The listing builds one solid part. Answer for the finished solid, in the listing's coordinates (mm). Face numbers are marked on the shaded views. A direction names the side the tool comes from. Coordinates: 2 decimals unless noted, no trailing zeros. Write each loop counter-clockwise with the first axis right and the second up, starting at its lowest first coordinate (ties: lowest second). Pieces come first, ordered by that corner, then holes.
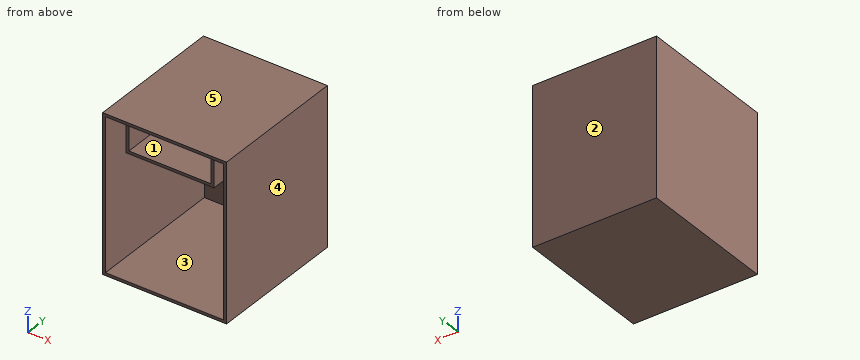
from build123d import *

# Parameters (mm, degrees)
F0_W     = 831.85
F0_H     = 1054.1
F0_W_2   = 793.75
F0_H_2   = 1016
F1_DEPTH = 914.4
F2_W     = 831.85
F2_H     = 1054.1
F3_DEPTH = 19.05
F6_DEPTH = 406.4


with BuildPart() as f1:
    # F0 (on Front) → F1 (new body)
    with BuildSketch(Plane.XZ):
        with Locations((396.875, 508)):
            Rectangle(F0_W, F0_H)
        with Locations((396.875, 508)):
            Rectangle(F0_W_2, F0_H_2, mode=Mode.SUBTRACT)
    extrude(amount=-F1_DEPTH)

    # F2 (on face) → F3 (join)
    with BuildSketch(Plane(origin=(0, 914.4, 0), x_dir=(-1, 0, 0), z_dir=(0, 1, 0))):
        with Locations((-396.875, 508)):
            Rectangle(F2_W, F2_H)
    extrude(amount=F3_DEPTH)

    # F5 (on offset) → F6 (join)
    with BuildSketch(Plane.XZ.offset(-50.8)):
        Polygon((120.65, 1016), (101.6, 1016), (101.6, 793.75), (692.15, 793.75), (692.15, 1016), (673.1, 1016), (673.1, 812.8), (120.65, 812.8), align=None)
    extrude(amount=-F6_DEPTH)


solid = f1.part
1. Section C-C on y = 560 is taken. Give the vertices of the cut face in (x, z).
Results found:
outline: (-19.05, -19.05) - (812.8, -19.05) - (812.8, 1035.05) - (-19.05, 1035.05) - close; hole (0, 0) - (793.75, 0) - (793.75, 1016) - (0, 1016) - close
2. Find the intervals of material crossed by L1, parallel to X at y = 161.5, z = 893; L2, parallel to Z at x = 322, y = 277; L3, parallel to Z at x = 282.5, y = 663, in increasing order.
Results found:
L1: x = -19.05 to 0, 101.6 to 120.65, 673.1 to 692.15, 793.75 to 812.8
L2: z = -19.05 to 0, 793.75 to 812.8, 1016 to 1035.05
L3: z = -19.05 to 0, 1016 to 1035.05
3. For a pull along X with two mould halves and no side action, classify the marked faces 3, 4 and 5 as pulls with the +X half, pulls with the -X half, needs draft (parallel to the pull), parting line crosses it, or undercut.
Results found:
face 3: undercut
face 4: pulls with the +X half
face 5: needs draft
4. A tool of negligible diameter and unlimited length cuts with its end or side. For the marked faces 1 and 2, from which of +Z, -Z, +X, -X, +Y, -Y can it reach the whole face along a straight path? Write none if from no direction.
Results found:
face 1: -Y
face 2: +Z, -Z, +X, -X, +Y
5. Section D-D on y = 406.5 is taken. Give the vertices of the cut face in (x, z), then the cut area to 3 significant figures.
Results found:
outline: (-19.05, -19.05) - (812.8, -19.05) - (812.8, 1035.05) - (-19.05, 1035.05) - close; hole (0, 0) - (793.75, 0) - (793.75, 1016) - (692.15, 1016) - (692.15, 793.75) - (101.6, 793.75) - (101.6, 1016) - (0, 1016) - close; hole (120.65, 812.8) - (673.1, 812.8) - (673.1, 1016) - (120.65, 1016) - close
area: 89,400 mm2
6. A flat-ended cylindrical pin translates along its axis: P1, Ø4, axis at x = 319.5, z = 845.5, coming from the -Y side. Find the tip coordinate at first contact, or state that the pin passes through.
Results found:
P1: stops at y = 914.4
7. Section A-A on z = 834 is taken. Give the vertices of the cut face in (x, y), then the cut area to 3 significant figures.
Results found:
outline: (-19.05, 0) - (0, 0) - (0, 914.4) - (793.75, 914.4) - (793.75, 0) - (812.8, 0) - (812.8, 933.45) - (-19.05, 933.45) - close; (101.6, 50.8) - (120.65, 50.8) - (120.65, 457.2) - (101.6, 457.2) - close; (673.1, 50.8) - (692.15, 50.8) - (692.15, 457.2) - (673.1, 457.2) - close
area: 66,200 mm2
8. Section B-B on x = 297.5 is taken. Give the vertices of the cut face in (y, z).
Results found:
outline: (0, -19.05) - (933.45, -19.05) - (933.45, 1035.05) - (0, 1035.05) - (0, 1016) - (914.4, 1016) - (914.4, 0) - (0, 0) - close; (50.8, 793.75) - (457.2, 793.75) - (457.2, 812.8) - (50.8, 812.8) - close
